Input: dimensioned drawing with shaded views. Units: mm. Origin: part minimum x, y, z. Give positions to 0.01 mm unless a question says otherwise; leave off trailing zeros. Write each loop counter-clockwise with the first axis right and the second up, starting at its lowest first coordinate (ties: lowest second). Pieces come first, ordered by that corner, then holes. Notation, with made-up numbers: (19, 17) -> (68, 17) arc R6 cw to (68, 24) -> close; hole circle Ø6 at (49.5, 53). An arc over 180 degrees is marked (long way). Return JSON: item names as keys, results as strings. Group by question number.
Item 1: Line query: line 1 (X direction, y = 1.55, z = 87.5); line 2 (Z direction, x = 23.25, y = 3); line 3 (X direction, y = 1.85, z = 67.5). Output: solid intervals per line, ascending. Write a range as [from, to].
Item 2: Pin query (flat end, axial travel): P1, Ø6, axis at x = 12, z = 53, coming from the -Y side. Return the tip coordinate at first contact, or that it passes through.
Item 3: Section A-A, the plane y = 1.55. Return loops of the section in (x, z).
Item 4: Section B-B, the plane z = 67.5. Return loops of the section in (x, y), then the cut area to 3 significant figures.
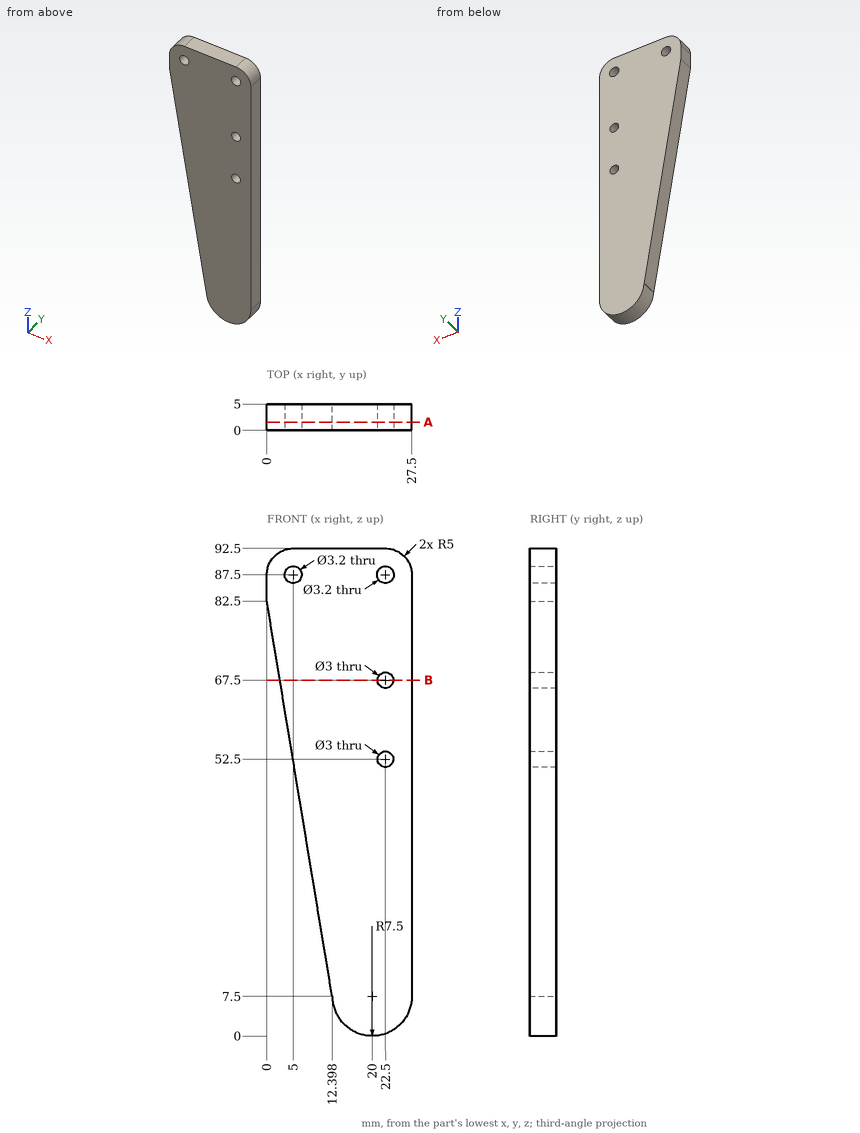
Answer below:
{
 "1": {"line 1": "x = [0, 3.4], [6.6, 20.9], [24.1, 27.5]", "line 2": "z = [0.74, 51.2], [53.8, 66.2], [68.8, 86.09], [88.91, 92.44]", "line 3": "x = [2.48, 21], [24, 27.5]"},
 "2": {"P1": "stops at y = 0"},
 "3": {"outline": "(0, 82.5) -> (12.4, 7.5) -> (12.5, 7.5) arc R7.5 ccw to (27.5, 7.5) -> (27.5, 87.5) arc R5 ccw to (22.5, 92.5) -> (5, 92.5) arc R5 ccw to (0, 87.5) -> close; hole circle Ø3.2 at (5, 87.5); hole circle Ø3.2 at (22.5, 87.5); hole circle Ø3 at (22.5, 52.5); hole circle Ø3 at (22.5, 67.5)"},
 "4": {"outline": "(2.48, 0) -> (21, 0) -> (21, 5) -> (2.48, 5) -> close; (24, 0) -> (27.5, 0) -> (27.5, 5) -> (24, 5) -> close", "area": "110 mm2"}
}
